Autodesk Inventor part; units mm, degrees
ref_plane "YZ Plane" through (0, 0, 0) normal (1, 0, 0) x (0, 1, 0)
ref_plane "XZ Plane" through (0, 0, 0) normal (0, 1, 0) x (-1, 0, 0)
ref_plane "XY Plane" through (0, 0, 0) normal (0, 0, 1) x (1, 0, 0)
sketch "Sketch1" plane through (0, 0, 0) normal (0, 0, 1) x (1, 0, 0)
  line L0 (-20.7464, 18.5829) -> (21.7536, 18.5829)
  line L1 (21.7536, 18.5829) -> (21.7536, -23.9171)
  line L2 (21.7536, -23.9171) -> (-20.7464, -23.9171)
  line L3 (-20.7464, -23.9171) -> (-20.7464, 18.5829)
  line L4 (-26.7464, 24.5829) -> (27.7536, 24.5829)
  line L5 (27.7536, 24.5829) -> (27.7536, -29.9171)
  line L6 (27.7536, -29.9171) -> (-26.7464, -29.9171)
  line L7 (-26.7464, -29.9171) -> (-26.7464, 24.5829)
  point P0 (0, 0)
  dimension "d0" = 42.5
  dimension "d1" = 42.5
  dimension "d2" = 6
  dimension "d3" = 6
  dimension "d4" = 6
  dimension "d5" = 6
extrude "Extrusion1" add sketch "Sketch1" along normal blind 30
chamfer "Chamfer1" distance 5 angle 45 4 edges at (27.7536, 24.5829, 15) (27.7536, -29.9171, 15) (21.7536, -23.9171, 15) (21.7536, 18.5829, 15)
chamfer "Chamfer2" distance 5 angle 45 2 edges at (-26.7464, 24.5829, 15) (-26.7464, -29.9171, 15)
sketch "Sketch2" plane through (22.7536, -29.9171, 0) normal (0, -1, 0) x (1, 0, 0)
  line L0 (-44.5, 30) -> (0, 30)
  point P0 (-22.7536, 0)
  point P1 (-22.7536, 15)
  dimension "d14" = 15
hole "Hole1" at (0, -29.9171, 15) direction (0, 1, 0) diameter 3 depth 100 tip angle 118
sketch "Sketch3" plane through (0, 0, 30) normal (0, 0, 1) x (1, 0, 0)
  line L0 (-21.7464, -29.9171) -> (22.7536, -29.9171)
  line L1 (-14.4964, -29.9171) -> (15.5036, -29.9171)
  line L2 (15.5036, -29.9171) -> (15.5036, -27.9171)
  line L3 (15.5036, -27.9171) -> (-14.4964, -27.9171)
  line L4 (-14.4964, -27.9171) -> (-14.4964, -29.9171)
  line L5 (-21.7464, 24.5829) -> (22.7536, 24.5829)
  line L6 (-14.4964, 24.5829) -> (15.5036, 24.5829)
  line L7 (15.5036, 24.5829) -> (15.5036, 22.5829)
  line L8 (15.5036, 22.5829) -> (-14.4964, 22.5829)
  line L9 (-14.4964, 22.5829) -> (-14.4964, 24.5829)
  line L10 (-20.7464, -23.9171) -> (-20.7464, 18.5829)
  point P0 (0, 0)
  dimension "d22" = 30
  dimension "d23" = 6.25
  dimension "d24" = 2
  dimension "d25" = 2
extrude "Extrusion2" cut sketch "Sketch3" against normal blind 30
sketch "Sketch4" plane through (-26.7464, -24.9171, 0) normal (-1, 0, 0) x (0, 0, 1)
  point P0 (0, 24.9171)
sketch "Sketch5" plane through (-26.7464, -24.9171, 0) normal (-1, 0, 0) x (0, 0, 1)
  line L0 (30, 38.5) -> (30, 6)
  line L1 (30, 34.1671) -> (0, 34.1671)
  line L2 (0, 34.1671) -> (0, 30.1671)
  line L3 (0, 30.1671) -> (30, 30.1671)
  line L4 (30, 30.1671) -> (30, 34.1671)
  line L5 (30, 19.6671) -> (0, 19.6671)
  line L6 (0, 19.6671) -> (0, 15.6671)
  line L7 (0, 15.6671) -> (30, 15.6671)
  line L8 (30, 15.6671) -> (30, 19.6671)
  line L9 (0, 0) -> (0, 44.5)
  point P0 (0, 24.9171)
  dimension "d28" = 10.5
  dimension "d29" = 4
  dimension "d30" = 4
  dimension "d31" = 5.25
extrude "Extrusion3" add sketch "Sketch5" along normal blind 10 contours L0 L3 L2 L1 | L0 L7 L6 L5
sketch "Sketch6" plane through (22.7536, -29.9171, 0) normal (0, -1, 0) x (1, 0, 0)
  point P0 (-22.7536, 0)
sketch "Sketch7" plane through (-14.4964, -27.9171, 30) normal (0, -1, 0) x (1, 0, 0)
  circle A0 centre (14.4964, -15) radius 1.5
  point P0 (14.4964, -30)
hole "Hole2" at (0, -27.9171, 15) direction (0, 1, 0) diameter 3 depth 100 tip angle 118 countersink diameter 6 countersink angle 90
sketch "Sketch8" plane through (-14.4964, 22.5829, 30) normal (0, 1, 0) x (1, 0, 0)
  circle A0 centre (14.4964, 15) radius 1.5
  point P0 (14.4964, 30)
hole "Hole3" at (0, 22.5829, 15) direction (0, -1, 0) diameter 3 depth 5 tip angle 118 countersink diameter 6 countersink angle 90
sketch "Sketch9" plane through (-26.7464, -9.25, 0) normal (0, -1, 0) x (1, 0, 0)
  line L0 (0, 30) -> (-10, 30)
  line L1 (0, 0) -> (-10, 0)
  point P0 (26.7464, 0)
  point P1 (-4.7181, 25)
  point P2 (-4.7181, 5)
  dimension "d48" = 5
  dimension "d49" = 5
hole "Hole4" at (-31.4645, -9.25, 25) at (-31.4645, -9.25, 5) direction (0, 1, 0) diameter 3 depth 5 tip angle 118 countersink diameter 6 countersink angle 90
sketch "Sketch10" plane through (-26.7464, 9.25, 30) normal (0, 1, 0) x (1, 0, 0)
  circle A0 centre (-4.7181, 5) radius 1.5
  circle A1 centre (-4.7181, 25) radius 1.5
  point P0 (26.7464, 30)
hole "Hole5" at (-31.4645, 9.25, 25) at (-31.4645, 9.25, 5) direction (0, -1, 0) diameter 3 depth 5 tip angle 118 countersink diameter 6 countersink angle 90
sketch "Sketch11" plane through (0, 0, 0) normal (0, 0, -1) x (-1, 0, 0)
  line L0 (-21.7536, 13.5829) -> (20.7464, 13.5829)
  line L1 (20.7464, 13.5829) -> (20.7464, 18.5829)
  line L2 (20.7464, 18.5829) -> (-21.7536, 18.5829)
  line L3 (-21.7536, 18.5829) -> (-21.7536, 13.5829)
  line L4 (20.7464, -23.9171) -> (-21.7536, -23.9171)
  line L5 (-21.7536, -23.9171) -> (-21.7536, -18.9171)
  line L6 (-21.7536, -18.9171) -> (20.7464, -18.9171)
  line L7 (20.7464, -18.9171) -> (20.7464, -23.9171)
  line L8 (20.7464, -23.9171) -> (-16.7536, -23.9171)
  point P0 (0, 0)
  dimension "d64" = 5
extrude "Extrusion4" add sketch "Sketch11" against normal blind 1.5
sketch "Sketch12" plane through (-26.7464, -5.25, 0) normal (-1, 0, 0) x (0, 0, 1)
  point P0 (0, 5.25)
sketch "Sketch13" plane through (-26.7464, -5.25, 0) normal (-1, 0, 0) x (0, 0, 1)
  line L0 (30, 10.5) -> (0, 10.5)
  line L1 (0, 10.5) -> (0, 0)
  line L2 (0, 0) -> (30, 0)
  line L3 (30, 0) -> (30, 10.5)
  point P0 (0, 5.25)
extrude "Extrusion5" cut sketch "Sketch13" against normal blind 6
chamfer "Chamfer3" distance 1 angle 45 1 edges at (-26.7464, 9.25, 15)
chamfer "Chamfer4" distance 1 angle 45 1 edges at (-26.7464, -9.25, 15)
properties part number "Stepper mount v1"
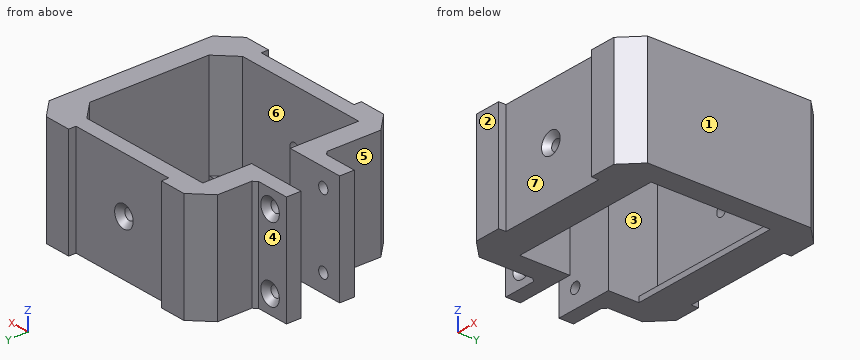
For this review, take the finished solid that the model builds, in its own axes (mm). Face numbers are marked on the shaded views. A direction names the side the tool comes from. Round coordinates to 2 decimals unless told otherwise and drop trailing zeros. Write each loop counter-clockwise with the first axis right and the second up, starting at its lowest first coordinate (ties: lowest second). Pieces come first, ordered by that corner, then holes. Notation, with made-up numbers: (4.5, 78) -> (53.5, 78) arc R18 ccw to (53.5, 95) -> close; hole circle Ø2 at (4, 35.5). An arc over 180 degrees is marked (long way). Put each result on its own line as item: value.
Q1. The part is to be moulded in two halves that separate along X. For the marked faces 1, 2 and 3, say which applies: released by +X, released by -X, zero draft, split by the parting line, or undercut.
Determined:
face 1: released by +X
face 2: zero draft
face 3: undercut
Q2. Clearance check with flat-ended pins moving along their axes: pin 1 Ø2.5 at (x, z) = (0, 15) entering from -Y; pin 2 Ø3.5 at (x, z) = (-31.46, 5) entering from -Y; pin 3 Ø4.5 at (y, z) = (14.5, 11) entering from -X; pin 4 Ø10 at (x, z) = (-31, 11.5) entering from -Y. State where each tip first meets the part, or that it passes through.
Determined:
pin 1: passes through
pin 2: stops at y = -8
pin 3: stops at x = -26.75
pin 4: stops at y = -25.66
Q3. Machinability: for the marked faces 4, 5, 6 and 7, which of the approach directions +Z, -Z, +X, -X, +Y, -Y give a long, thin tool a straight path to every point of the face, cutting with its end or side? Answer none if there is none.
Determined:
face 4: +Z, -Z, -X, +Y
face 5: +Z, -Z, -X, -Y
face 6: +Z
face 7: +Z, -Z, -Y
Q4. Consider section B-B on y = 12. State the section outline as (x, z) points.
Determined:
outline: (-26.75, 0) -> (-20.75, 0) -> (-20.75, 30) -> (-26.75, 30) -> close; (21.75, 0) -> (27.75, 0) -> (27.75, 30) -> (21.75, 30) -> close
Q5. To check wall thickness, follow L1, parallel to X at y = 7, z = 5; L2, parallel to Y at x = -19, z = 26.25; L3, parallel to Y at x = -6.5, z = 9.5. State the ranges of each line that lie inside material, in increasing order. Write a range as [from, to].
Determined:
L1: x = [-36.75, -32.96], [-29.96, -20.75], [21.75, 27.75]
L2: y = [-29.92, -23.92], [18.58, 24.58]
L3: y = [-27.92, -23.92], [18.58, 22.58]
Q6. Consider section C-C on z = 15. Give the number of separate pieces and of enclosed holes in the cut face, and give its area (3 significant figures).
Determined:
separate pieces: 3
enclosed holes: 0
area: 1,010 mm^2
Q7. Consider section A-A on x = -16.5. State the section outline as (y, z) points.
Determined:
outline: (-29.92, 0) -> (-18.92, 0) -> (-18.92, 1.5) -> (-23.92, 1.5) -> (-23.92, 30) -> (-29.92, 30) -> close; (13.58, 0) -> (24.58, 0) -> (24.58, 30) -> (18.58, 30) -> (18.58, 1.5) -> (13.58, 1.5) -> close
Q8. Consider section D-D on x = -4. State the section outline as (y, z) points, and give its area (3 significant figures).
Determined:
outline: (-27.92, 0) -> (-18.92, 0) -> (-18.92, 1.5) -> (-23.92, 1.5) -> (-23.92, 30) -> (-27.92, 30) -> close; (13.58, 0) -> (22.58, 0) -> (22.58, 30) -> (18.58, 30) -> (18.58, 1.5) -> (13.58, 1.5) -> close
area: 255 mm^2
